Design review of the part shown in the three views and the two pictorial views. Dimensions are in mm from the part's minimum x, y and z. A direction names the side the tool comes from. Coordinates: 2 decimals unless noted, no trailing zeros. Loops run counter-clockwise (first coordinate to the right, second up) from the corner with the lowest first, then second, coordinate; pieces in that order, holes last. Notation, with made-up numbers: (-38.75, 58.5) -> (-20.75, 58.5) arc R23 ccw to (-20.75, 96.5) -> close; hole circle Ø10 at (85, 39.25). An arc over 180 degrees is marked (long way). Answer in a Markdown table with one row per item.
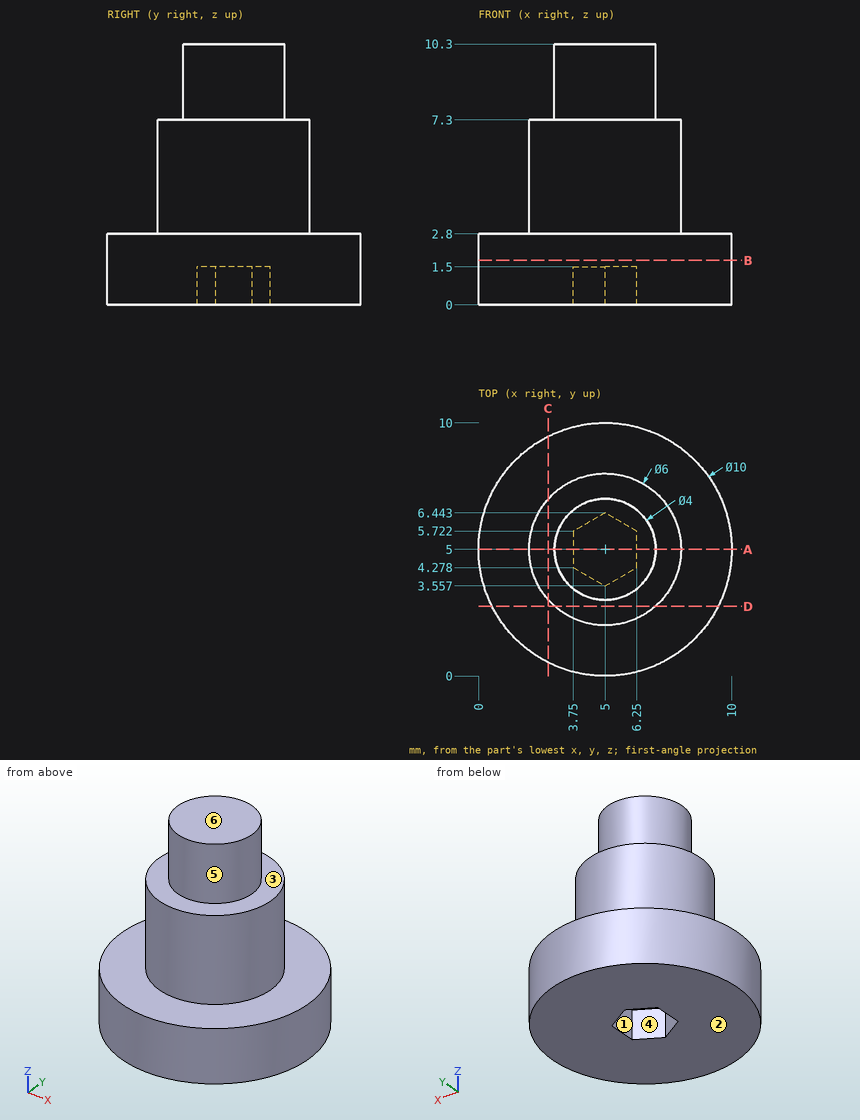
Item 1: Insertion check: pin 1 (2 mm diameter, centred on x = 8, y = 2, fed in from -Z); pin 2 (2 mm diameter, centred on x = 5, y = 5, fed in from -Z); pin 3 (4 mm diameter, centred on x = 8.5, y = 1.5, fed in from +Z); pin 4 (1.5 mm diameter, centred on y = 9, z = 5, fed in from +X). Each pin has a flat end and moves straight along its axis. Give the tip position at first contact, or say it passes through.
Worked answers:
| item | result |
|---|---|
| pin 1 | z = 0 |
| pin 2 | z = 1.5 |
| pin 3 | z = 7.3 |
| pin 4 | through |
Item 2: For the marked faces 1, 2 and 3, list the 3-axis set-ups (+Z, -Z, +X, -X, +Y, -Y) from which the entire face can be reached by the end or side of a thin tool; tool diameter is ignored.
Worked answers:
| item | result |
|---|---|
| face 1 | -Z |
| face 2 | -Z, +X, -X, +Y, -Y |
| face 3 | +Z |
Item 3: The part is to be moulded in two halves that separate along Y. For the marked faces 4, 5 and 6, say which applies: +Y half, -Y half, draft (parallel to the pull), parting line (faces both ways), or undercut.
Worked answers:
| item | result |
|---|---|
| face 4 | undercut |
| face 5 | parting line |
| face 6 | draft |
Item 4: Take a section at A-A, the plane y = 5. State the section outline as (x, z) points.
Worked answers:
| item | result |
|---|---|
| outline | (0, 0) -> (3.75, 0) -> (3.75, 1.5) -> (6.25, 1.5) -> (6.25, 0) -> (10, 0) -> (10, 2.8) -> (8, 2.8) -> (8, 7.3) -> (7, 7.3) -> (7, 10.3) -> (3, 10.3) -> (3, 7.3) -> (2, 7.3) -> (2, 2.8) -> (0, 2.8) -> close |
Item 5: Take a section at C-C, the plane x = 2.75. State the section outline as (y, z) points (1 decimal).
Worked answers:
| item | result |
|---|---|
| outline | (0.5, 0) -> (9.5, 0) -> (9.5, 2.8) -> (7, 2.8) -> (7, 7.3) -> (3, 7.3) -> (3, 2.8) -> (0.5, 2.8) -> close |
Item 6: For L1, parallel to Z at x = 3, y = 2.25; L2, parallel to Z at x = 5, y = 4; L3, parallel to Y at x = 3.5, z = 4.5, list the stretches that pass through material, from the lowest coordinate up.
Worked answers:
| item | result |
|---|---|
| L1 | 0 to 2.8 |
| L2 | 1.5 to 10.3 |
| L3 | 2.4 to 7.6 |
Item 7: Take a section at B-B, the plane z = 1.75. State the section outline as (x, y) points.
Worked answers:
| item | result |
|---|---|
| outline | circle Ø10 at (5, 5) |
